from build123d import *

# Parameters (mm, degrees)
SKETCH1_R           = 1.55
BOSS_EXTRUDE1_DEPTH = 1.6
SKETCH2_W           = 6.9
SKETCH2_H           = 7.5
BOSS_EXTRUDE2_DEPTH = 8.8
SKETCH3_R           = 4.1
BOSS_EXTRUDE3_DEPTH = 12.9
SKETCH4_W           = 7.5
SKETCH4_H           = 10
BOSS_EXTRUDE4_DEPTH = 2.75
SKETCH6_W           = 17.5
SKETCH6_H           = 5.8
BOSS_EXTRUDE5_DEPTH = 7


with BuildPart() as part:
    # Sketch1 → Boss-Extrude1 (new body)
    with BuildSketch(Plane(origin=(0, 0, 0), x_dir=(1, 0, 0), z_dir=(0, 1, 0))):
        with BuildLine():
            Line((3, 0), (22.5, 0))
            ThreePointArc((22.5, 0), (24.621320344, 0.878679656), (25.5, 3))
            Line((25.5, 3), (25.5, 59.2))
            ThreePointArc((25.5, 59.2), (24.621320344, 61.321320344), (22.5, 62.2))
            Line((22.5, 62.2), (3, 62.2))
            ThreePointArc((3, 62.2), (0.878679656, 61.321320344), (0, 59.2))
            Line((0, 59.2), (0, 3))
            ThreePointArc((0, 3), (0.878679656, 0.878679656), (3, 0))
        make_face()
        with Locations((3, 59.2)):
            Circle(SKETCH1_R, mode=Mode.SUBTRACT)
        with Locations((22.5, 59.2)):
            Circle(SKETCH1_R, mode=Mode.SUBTRACT)
        with Locations((22.5, 3)):
            Circle(SKETCH1_R, mode=Mode.SUBTRACT)
        with Locations((3, 3)):
            Circle(SKETCH1_R, mode=Mode.SUBTRACT)
    extrude(amount=BOSS_EXTRUDE1_DEPTH)

    # Sketch2 → Boss-Extrude2 (add)
    with BuildSketch(Plane(origin=(0, 1.6, 0), x_dir=(1, 0, 0), z_dir=(0, 1, 0))):
        with Locations((3.65, 31)):
            Rectangle(SKETCH2_W, SKETCH2_H)
    extrude(amount=BOSS_EXTRUDE2_DEPTH)

    # Sketch3 → Boss-Extrude3 (add)
    with BuildSketch(Plane(origin=(0, 1.6, 0), x_dir=(1, 0, 0), z_dir=(0, 1, 0))):
        with Locations((4.3, 12.75)):
            Circle(SKETCH3_R)
    extrude(amount=BOSS_EXTRUDE3_DEPTH)

    # Sketch4 → Boss-Extrude4 (add)
    with BuildSketch(Plane(origin=(0, 1.6, 0), x_dir=(1, 0, 0), z_dir=(0, 1, 0))):
        with Locations((21.55, 10.8)):
            Rectangle(SKETCH4_W, SKETCH4_H)
        with Locations((21.55, 23.3)):
            Rectangle(SKETCH4_W, SKETCH4_H)
        with Locations((21.55, 38.9)):
            Rectangle(SKETCH4_W, SKETCH4_H)
        with Locations((21.55, 51.4)):
            Rectangle(SKETCH4_W, SKETCH4_H)
    extrude(amount=BOSS_EXTRUDE4_DEPTH)

    # Sketch6 → Boss-Extrude5 (add)
    with BuildSketch(Plane(origin=(0, 1.6, 0), x_dir=(1, 0, 0), z_dir=(0, 1, 0))):
        with Locations((12.75, 2.9)):
            Rectangle(SKETCH6_W, SKETCH6_H)
    extrude(amount=BOSS_EXTRUDE5_DEPTH)


solid = part.part
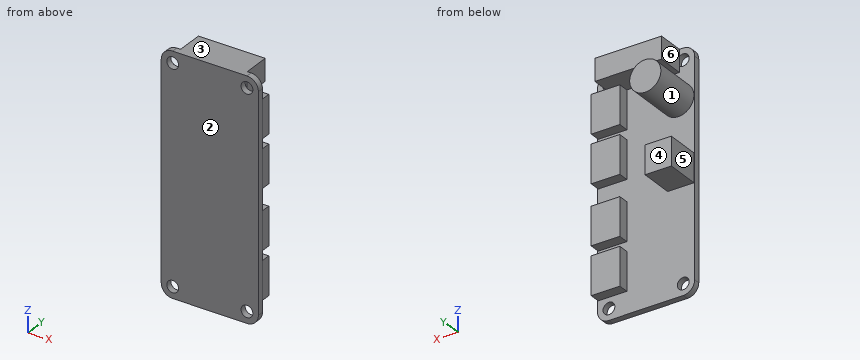
The model under review builds one solid part; all positions refer to its coordinate system, in mm. Face numbers are marked on the shaded views. A direction names the side the tool comes from. Round coordinates to 2 decimals unless told otherwise and drop trailing zeros. Order: outer loops, then holes, each group sorted by start corner. A loop starts at its lowest first (then second) coordinate and runs counter-clockwise, first axis right, second up. Notation, with made-up numbers: (54.25, -14) -> (113.25, -14) arc R26 cw to (113.25, 14) -> close; hole circle Ø11 at (21.5, 85.25). An arc over 180 degrees is marked (long way). Return JSON: item names as keys, results as strings.
1. For the marked faces 4, 5 and 6, list the 3-axis set-ups (+Z, -Z, +X, -X, +Y, -Y) from which the entire face can be reached by the end or side of a thin tool; tool diameter is ignored.
Answer block:
{"face 4": "-Z, +X, -X, +Y", "face 5": "+Z, -Z, -X, +Y", "face 6": "+Z, -X, +Y"}
2. Insertion check: P1, Ø6, axis at y = 6, z = -47.5, coming from the -X side; P2, Ø1.9, axis at x = 22.5, z = -3, coming from the -Y side; P3, Ø6, axis at x = 22, z = -53, coming from the +Y side; P4, Ø4, axis at y = 4.5, z = -32, coming from the +X side. Each pin has a flat end and moves straight along its axis. Give the tip position at first contact, or say it passes through.
Answer block:
{"P1": "stops at x = 17.8", "P2": "passes through", "P3": "stops at y = 4.35", "P4": "stops at x = 25.3"}
3. The part is to be moulded in two halves that separate along Z. For the marked faces 1, 2 and 3, say which applies: +Z half, -Z half, draft (parallel to the pull), parting line (faces both ways), or undercut.
Answer block:
{"face 1": "undercut", "face 2": "draft", "face 3": "+Z half"}
4. Take a section at B-B (z = -33). Write out the cut boundary in (x, y).
Answer block:
{"outline": "(0, 0) -> (25.5, 0) -> (25.5, 1.6) -> (7.1, 1.6) -> (7.1, 10.4) -> (0.2, 10.4) -> (0.2, 1.6) -> (0, 1.6) -> close"}
5. For L1, parallel to X at y = 1.1, z = -59.2; L2, parallel to Z at x = 22.5, y = 0.75; L3, parallel to Z at x = 20.5, y = 3.75, list the stretches that pass through material, from the lowest coordinate up. Write a range as [from, to].
Answer block:
{"L1": "x = [0, 1.45], [4.55, 20.95], [24.05, 25.5]", "L2": "z = [-62.2, -60.75], [-57.65, -4.55], [-1.45, 0]", "L3": "z = [-56.4, -46.4], [-43.9, -33.9], [-28.3, -18.3], [-15.8, 0]"}
6. Take a section at A-A (y = 3). Write out the cut boundary in (x, z), then the cut area to 3 significant figures.
Answer block:
{"outline": "(0.2, -34.75) -> (7.1, -34.75) -> (7.1, -27.25) -> (0.2, -27.25) -> close; circle Ø8.2 at (4.3, -12.75); (4, -5.8) -> (17.8, -5.8) -> (17.8, -15.8) -> (25.3, -15.8) -> (25.3, -5.8) -> (21.5, -5.8) -> (21.5, 0) -> (4, 0) -> close; (17.8, -56.4) -> (25.3, -56.4) -> (25.3, -46.4) -> (17.8, -46.4) -> close; (17.8, -43.9) -> (25.3, -43.9) -> (25.3, -33.9) -> (17.8, -33.9) -> close; (17.8, -28.3) -> (25.3, -28.3) -> (25.3, -18.3) -> (17.8, -18.3) -> close", "area": "506 mm²"}
7. Take a section at C-C (x = 9.25). Write out the cut boundary in (y, z), then the cut area to 3 significant figures.
Answer block:
{"outline": "(0, -62.2) -> (1.6, -62.2) -> (1.6, -5.8) -> (8.6, -5.8) -> (8.6, 0) -> (0, 0) -> close", "area": "140 mm²"}
8. Take a section at D-D (z = -47.5). Write out the cut boundary in (x, y), then the cut area to 3 significant figures.
Answer block:
{"outline": "(0, 0) -> (25.5, 0) -> (25.5, 1.6) -> (25.3, 1.6) -> (25.3, 4.35) -> (17.8, 4.35) -> (17.8, 1.6) -> (0, 1.6) -> close", "area": "61.4 mm²"}
